Print and shaded views of the part. All mm, measured from the part's lowest x, y and z. A direction names the side the tool comes from. Coordinates: 2 decimals unless noted, no trailing zeros. Loops run counter-clockwise (first coordinate to the right, second up) from the corner with the lowest first, then second, coordinate; pieces in that order, holes last. Notation, with made-up numbers: M 8.5,21.5 L 50.5,21.5 A20 ccw 50.5,44.5 Z; hole C -8,13 d9. An arc over 180 degrees is marked long. Answer as CSV lines item,"result". Start each with the question number.
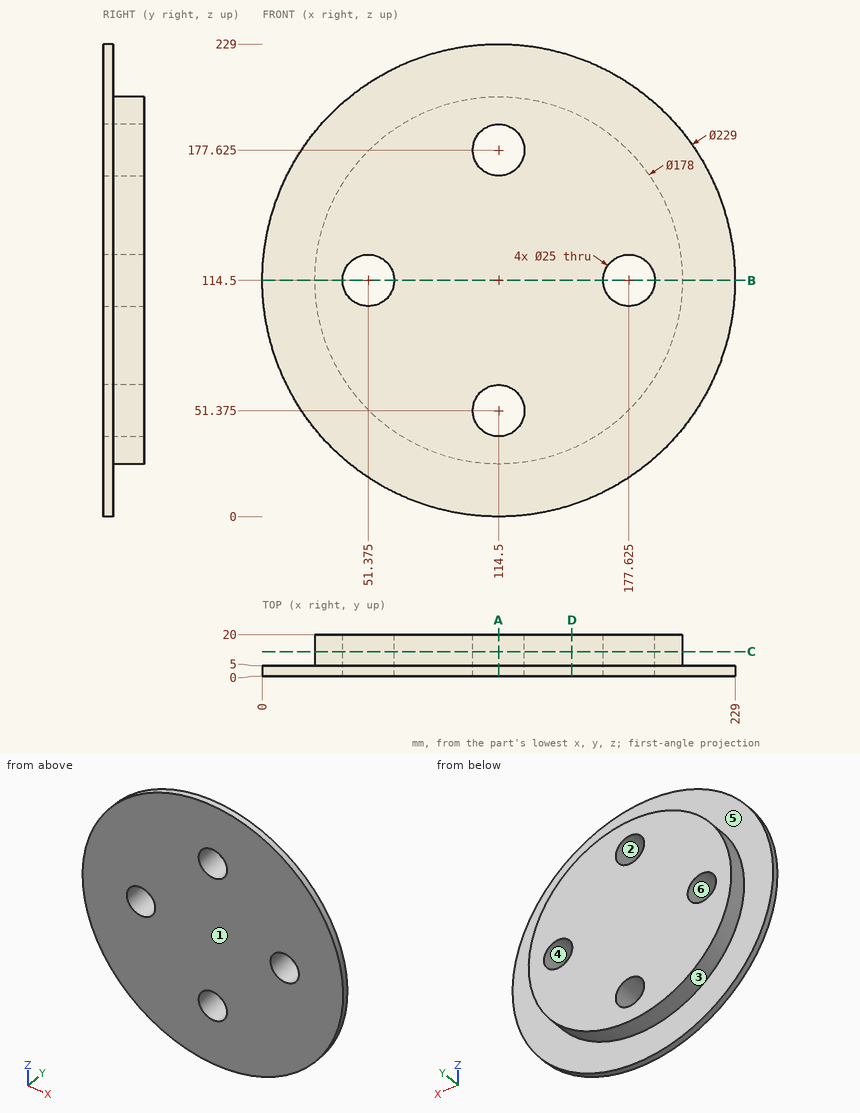
Q1. Slice it at D-D, the plane x = 150. Write the cut outline in (y, z), and give its area (3 significant figures).
Q2. Wall check: L1, parallel to X at y = 6, z = 114.5 (3 decimals); L2, parallel to Y at x = 28.5, z = 143; L3, parallel to Z at x = 108, y = 6.25. Give the ranges that are in metal, low to high.
Q3. Flat gauge pins, fed straight in: P1, Ø15, axis at x = 114.5, z = 177.62, coming from the -Y side; P2, Ø6, axis at x = 24, y = 7, coming from the -Z side; P3, Ø10, axis at y = 7, z = 170.5, coming from the -X side; P4, Ø12, axis at x = 173, y = 17, coming from the -Z side. Where does each tip first touch, or does it go through?
Q4. Tool access for the marked faces 5 and 6: list every direction of +Z, -Z, +X, -X, +Y, -Y with a clear straight run to the whole face (end or side of a thin tool).
Q5. Slice it at A-A, the plane x = 114.5. Write the cut outline in (y, z) (3 decimals), and give its area (4 significant figures).
Q6. Slice it at B-B, the plane z = 114.5. Write the cut outline in (x, y) (3 decimals).
Q7. Slice it at C-C, the plane y = 11.75. Write the cut outline in (x, z) (3 decimals).
Q8. Two-plate mould, pull along Z, no slides. Class the marked faces 1, 2, 3 and 4: +Z half, -Z half, draft (parallel to the pull), parting line (faces both ways), or undercut.
Solved:
1,outline,"M 0,5.64 L 5,5.64 L 5,32.89 L 20,32.89 L 20,196.11 L 5,196.11 L 5,223.36 L 0,223.36 Z"
1,area,"3,540 mm2"
2,L1,"x = 25.5 to 38.875, 63.875 to 165.125, 190.125 to 203.5"
2,L2,"y = 0 to 5"
2,L3,"z = 25.74 to 40.7, 62.05 to 166.95, 188.3 to 203.26"
3,P1,"passes through"
3,P2,"stops at z = 41.56"
3,P3,"stops at x = 12.19"
3,P4,"stops at z = 42.63"
4,face 5,"+Y"
4,face 6,"+Y, -Y"
5,outline,"M 0,0 L 5,0 L 5,25.5 L 20,25.5 L 20,38.875 L 0,38.875 Z; M 0,63.875 L 20,63.875 L 20,165.125 L 0,165.125 Z; M 0,190.125 L 20,190.125 L 20,203.5 L 5,203.5 L 5,229 L 0,229 Z"
5,area,"2,815 mm2"
6,outline,"M 0,0 L 38.875,0 L 38.875,20 L 25.5,20 L 25.5,5 L 0,5 Z; M 63.875,0 L 165.125,0 L 165.125,20 L 63.875,20 Z; M 190.125,0 L 229,0 L 229,5 L 203.5,5 L 203.5,20 L 190.125,20 Z"
7,outline,"C 114.5,114.5 d178; hole C 51.375,114.5 d25; hole C 114.5,51.375 d25; hole C 114.5,177.625 d25; hole C 177.625,114.5 d25"
8,face 1,"draft"
8,face 2,"undercut"
8,face 3,"parting line"
8,face 4,"undercut"
